For this review, take the finished solid that the model builds, in its own axes (mm). Face numbers are marked on the shaded views. Coordinates: 2 decimals unless noted, no trailing zeros. Loops run counter-clockwise (first coordinate to the right, second up) from the corner with the lowest first, then second, coordinate; pieces in that order, holes last. Notation, with made-up numbers: M 57.25,-40 L 92.25,-40 A32 cw 92.25,-14 Z; hole C 34,69 d9. An arc over 180 degrees is marked long. Write item = value, one per line.
Autodesk Fusion 360 part; units mm, degrees
sketch "base" plane through (0, 0, 0) normal (0, 0, 1) x (1, 0, 0)
  line L0 (-20, 30) -> (20, 30)
  line L1 (30, 20) -> (30, -20)
  line L2 (20, -30) -> (-20, -30)
  line L3 (-30, -20) -> (-30, 20)
  line L4 (-30, 30) -> (30, -30) construction
  line L5 (30, 30) -> (-30, -30) construction
  arc A0 (-20, 30) -> (-30, 20) centre (-20, 20) ccw
  arc A1 (30, 20) -> (20, 30) centre (20, 20) ccw
  arc A2 (20, -30) -> (30, -20) centre (20, -20) ccw
  arc A3 (-30, -20) -> (-20, -30) centre (-20, -20) ccw
  dimension "d1" = 10
  dimension "d2" = 40
  dimension "d3" = 40
extrude "Extrude1" add sketch "base" along normal blind 5
sketch "post anchor" plane through (0, 0, 5) normal (0, 0, 1) x (-1, 0, 0)
  arc A0 (20, -30) -> (30, -20) centre (20, -20) ccw
  line L0 (30, -20) -> (30, 20)
  arc A1 (30, 20) -> (20, 30) centre (20, 20) ccw
  line L1 (20, 30) -> (-20, 30)
  arc A2 (-20, 30) -> (-30, 20) centre (-20, 20) ccw
  line L2 (-30, 20) -> (-30, -20)
  arc A3 (-30, -20) -> (-20, -30) centre (-20, -20) ccw
  line L3 (-20, -30) -> (20, -30)
  line L4 (4.7066, -30) -> (-5.2934, -30)
  line L5 (4.7066, -30) -> (4.7066, -20)
  line L6 (4.7066, -20) -> (-5.2934, -20)
  line L7 (-5.2934, -20) -> (-5.2934, -30)
  point P0 (0, -30)
  dimension "d6" = 10
  dimension "d7" = 10
extrude "Extrude2" add sketch "post anchor" along normal blind 57 contours L3 L4 L5 L6 L7
sketch "stand profile" plane through (5.2934, 0, 0) normal (1, 0, 0) x (0, 1, 0)
  line L0 (20, 5) -> (30, 5)
  line L1 (30, 5) -> (30, 62)
  line L2 (30, 62) -> (20, 62)
  line L3 (20, 62) -> (20, 5)
  line L4 (20, 5) -> (30, 5)
  line L5 (30, 62) -> (20, 62)
  line L6 (20, 59.97) -> (24.4513, 59.97)
  line L7 (26.4513, 57.97) -> (26.4513, 7.6053)
  line L8 (26.4513, 7.6053) -> (20, 7.6053)
  line L9 (20, 5) -> (20, 7.6053)
  line L10 (20, 62) -> (20, 59.97)
  arc A0 (26.4513, 57.97) -> (24.4513, 59.97) centre (24.4513, 57.97) ccw
  dimension "d10" = 3.5487
  dimension "d11" = 2.6053
  dimension "d12" = 2.03
  dimension "d13" = 2
extrude "Extrude3" cut sketch "stand profile" against normal blind 10 contours L3 L6 L7 L8 A0
sketch "headphone rest" plane through (5.2934, 0, 0) normal (1, 0, 0) x (0, 1, 0)
  line L0 (26.4513, 7.6053) -> (20, 7.6053)
  line L1 (20, 7.6053) -> (20, 5)
  line L2 (20, 5) -> (30, 5)
  line L3 (30, 5) -> (30, 62)
  line L4 (30, 62) -> (20, 62)
  line L5 (20, 62) -> (20, 59.97)
  line L6 (20, 59.97) -> (24.4513, 59.97)
  arc A0 (26.4513, 57.97) -> (24.4513, 59.97) centre (24.4513, 57.97) ccw
  line L7 (26.4513, 57.97) -> (26.4513, 7.6053)
  line L8 (21, 62) -> (21, 61)
  line L9 (21, 61) -> (29, 61)
  line L10 (29, 61) -> (29, 62)
  line L11 (30, 62) -> (30, 60.477)
  line L12 (20, 60.477) -> (20, 62)
  line L13 (21, 62) -> (20, 62)
  line L14 (20, 60.477) -> (30, 60.477)
  dimension "d16" = 1
  dimension "d17" = 1
  dimension "d18" = 0.523
  dimension "d19" = 1
extrude "Extrude4" cut sketch "headphone rest" against normal blind 10 contours L4 L8 L9 L10
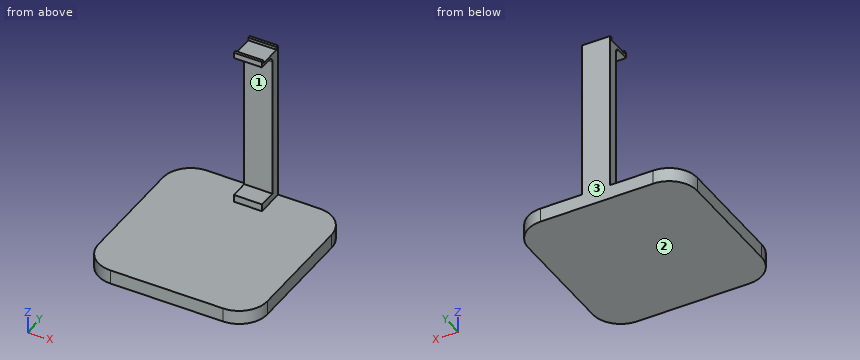
Q1. Add section C-C (z = 41). Write out the cut boundary in (x, y), and give its area (3 significant figures).
Solved:
outline = M -4.71,26.45 L 5.29,26.45 L 5.29,30 L -4.71,30 Z
area = 35.5 mm²
Q2. Draft analysis for pull direction Z (two halves, no side actions). For the marked faces 1, 2 and 3, state which applies: +Z half, -Z half, draft (parallel to the pull), parting line (faces both ways), or undercut.
Solved:
face_1 = undercut
face_2 = -Z half
face_3 = draft
Q3. Add section D-D (y = -15). Write out the cut boundary in (x, z), and give its area (3 significant figures).
Solved:
outline = M -30,0 L 30,0 L 30,5 L -30,5 Z
area = 300 mm²
Q4. Add section A-A (x = 0.5). Write out the cut boundary in (y, z).
Solved:
outline = M -30,0 L 30,0 L 30,62 L 29,62 L 29,61 L 21,61 L 21,62 L 20,62 L 20,59.97 L 24.45,59.97 A2 cw 26.45,57.97 L 26.45,7.61 L 20,7.61 L 20,5 L -30,5 Z
Q5. For pin 1 Ø4 at (x, y) = (2.5, 23.5) entering from +Z; pin 2 Ø8 at (x, z) = (1, 25) entering from -Y; pin 3 Ø3 at (y, z) = (25.5, 21.5) entering from +X, all flat-tipped, find the tip position at first contact; note any pin that passes through.
Solved:
pin_1 = 61
pin_2 = 26.45
pin_3 = 5.29
Q6. For line 1 along Z through (x, y) = (-7.5, 22.5); line 2 along Y through (x, z) = (3.5, 24.5), list the stretches that pass through material, from the lowest coordinate up.
Solved:
line_1 = 0 to 5
line_2 = 26.45 to 30
Q7. Add section B-B (y = 22.5). Write out the cut boundary in (x, z), and give its area (3 significant figures).
Solved:
outline = M -29.68,0 L 29.68,0 L 29.68,5 L 5.29,5 L 5.29,7.61 L -4.71,7.61 L -4.71,5 L -29.68,5 Z; M -4.71,59.97 L 5.29,59.97 L 5.29,61 L -4.71,61 Z
area = 333 mm²
